Work out the finished part from the listing and answer in its coordinate system (mm). Face numbers are marked on the shaded views. A direction names the side the tool comes from. Round coordinates to 2 decimals unless told otherwise and drop trailing zeros. Order: outer loops, then holes, each group sorted by start corner. A loop starts at its lowest first (then second) coordinate and runs counter-clockwise, first axis right, second up. Notation, with made-up numbers: (75.5, -21) - (96.5, -21) arc R29 cw to (96.5, 16) - close; hole circle Ø10 at (-29.5, 43). An arc over 180 degrees is marked (long way). Put each result on its own line as item: value.
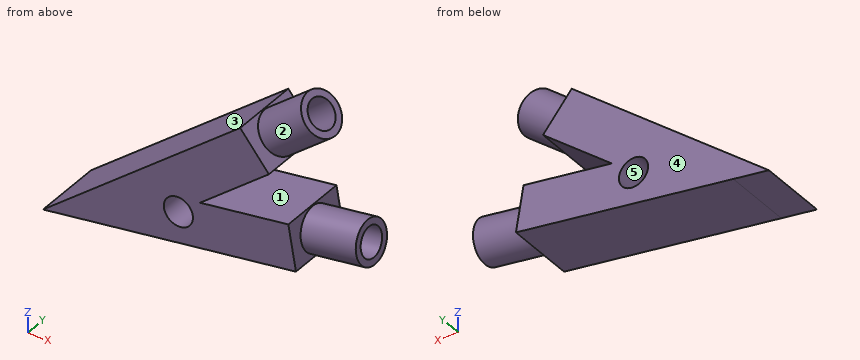
```python
from build123d import *

# Parameters (mm, degrees)
F0_R     = 6.50875
F1_DEPTH = 30
F3_R     = 9.4868068264
F3_R_2   = 6.50875
F4_DEPTH = 25
F2_R     = 9.5596537672
F2_R_2   = 6.50875
F5_DEPTH = 25


with BuildPart() as f1:
    # F0 (on Front) → F1 (new body)
    with BuildSketch(Plane.XZ):
        Polygon((-0.6586156459, -22.1222693219), (-40.0733649731, -28.9397127926), (-9.3479125073, -3.3282588946), (-22.1536394563, 12.0344673383), (-110.213566766, -61.3686101614), (-94.3012574901, -58.6163087811), (2.7501060895, -41.8296439855), align=None)
        with Locations((-49.7683258624, -37.0436192746)):
            Circle(F0_R, mode=Mode.SUBTRACT)
    extrude(amount=F1_DEPTH)

    # F3 (on face) → F4 (join)
    with BuildSketch(Plane(origin=(-4.3547506781, 0, -0.7532273345), x_dir=(0, 1, 0), z_dir=(0.9853687332, 0, 0.1704360868))):
        with Locations((-15, -31.6863406234)):
            Circle(F3_R)
        with Locations((-15, -31.6863406234)):
            Circle(F3_R_2, mode=Mode.SUBTRACT)
    extrude(amount=F4_DEPTH)

    # F2 (on face) → F5 (join)
    with BuildSketch(Plane(origin=(-7.1525087674, 0, -5.9620325773), x_dir=(0, 1, 0), z_dir=(0.7681363116, 0, 0.6402863475))):
        with Locations((-15, 13.4287842441)):
            Circle(F2_R)
        with Locations((-15, 13.4287842441)):
            Circle(F2_R_2, mode=Mode.SUBTRACT)
    extrude(amount=F5_DEPTH)


solid = f1.part
```
1) For a pull along Z with two mould halves and no side action, classify the marked faces 3, 4 and 5 as pulls with the +Z half, pulls with the -Z half, needs draft (parallel to the pull), parting line crosses it, or undercut.
Findings below:
face 3: pulls with the +Z half
face 4: needs draft
face 5: undercut
2) A cutting plane is placed at D-D on z = -10.5. Write down the section's boundary in (x, y).
Findings below:
outline: (-49.19, -30) - (-17.95, -30) - (-17.95, 0) - (-49.19, 0) - close
3) A cutting plane is placed at A-A on x = -48. Write down the section's boundary in (y, z).
Findings below:
outline: (-30, -50.61) - (0, -50.61) - (0, -43.31) - (-30, -43.31) - close; (-30, -30.78) - (0, -30.78) - (0, -9.51) - (-30, -9.51) - close
4) For the marked faces 1 and 2, determine the directions among +Z, -Z, +X, -X, +Y, -Y from which every point of the face is accessible in a straight line to the end or side of a thin tool.
Findings below:
face 1: +Y, -Y
face 2: none
5) A cutting plane is placed at C-C on x = -14. Give the number of separate pieces and of enclosed holes in the cut face, then the cut area to 3 significant figures.
Findings below:
separate pieces: 2
enclosed holes: 1
area: 1,020 mm2
6) Given pin 1 Ø6 at (x, y) = (-61.5, -14) entering from -Z; pin 2 Ø5 at (x, y) = (1.5, -11) entering from +Z; pin 3 Ø6 at (x, y) = (-34.5, -22.5) entering from -Z, each flat-ended and moving along its own axis, determine where each tip first touches the part or whether it passes through.
Findings below:
pin 1: stops at z = -53.46
pin 2: stops at z = 25.7
pin 3: stops at z = -48.79
7) A cutting plane is placed at B-B on y = -11. Write down the section's boundary in (x, z).
Findings below:
outline: (-110.21, -61.37) - (2.75, -41.83) - (2.51, -40.45) - (27.15, -36.19) - (26.56, -32.77) - (1.92, -37.04) - (0.17, -26.92) - (24.8, -22.66) - (24.21, -19.24) - (-0.42, -23.5) - (-0.66, -22.12) - (-40.07, -28.94) - (-9.35, -3.33) - (-10.19, -2.32) - (9.01, 13.69) - (6.74, 16.42) - (-12.46, 0.41) - (-19.04, 8.3) - (0.17, 24.3) - (-2.11, 27.03) - (-21.31, 11.02) - (-22.15, 12.03) - close; hole circle Ø13.02 at (-49.77, -37.04)
8) Straight lines are drawn through the part: L1, parallel to Z at x = -30.5, y = -13; L2, parallel to Z at x = -4, y = -14.25; L3, parallel to Z at x = -34.5, y = -24.75. For each, find the intervals that lie inside material, in ascending order. Write a range as from..to.
Findings below:
L1: z = -47.58..-27.28, -20.96..5.08
L2: z = -43..-22.7, 1.74..5.73, 22.57..26.55
L3: z = -48.27..-27.98, -24.29..1.74
